Job drawing, mm, ordinate dimensions from the low corner. One solid piece. Give positions to 0.01 mm unless a question says otherwise; leave off trailing zeros. Order: outer loops, then holes, each group sorted by start corner. A loop starts at its lowest first (then second) coordinate and runs counter-clockwise, first axis right, second up.
Item 1: Band-saw the part on B-B on y = 72. Give the cut face in (x, z).
Item 2: Band-saw the part on C-C on x = 23.5. Give the cut face in (y, z), plus the area to 3 significant figures.
Item 3: Band-saw the part on D-D on z = 2.4. Give the cut face in (x, y).
Item 4: Flat gauge pins, fed straight in: P1, Ø1, axis at y = 25.5, z = 2, coming from the +X side; P2, Ø8, axis at x = 72, y = 72, coming from the -Z side; P3, Ø1.5, axis at y = 30, z = 2, coming from the +X side. Where does each tip first touch, or does it go through?
Item 5: Wall check: L1, parallel to Y at x = 72, z = 1.6; L2, parallel to Y at x = 27.5, z = 1.5; L3, parallel to X at y = 51.5, z = 2.9. Give the ranges that are in metal, low to high.
Item 6: Band-saw the part on A-A on x = 72. Give the cut face in (y, z), plus the area to 3 significant figures.
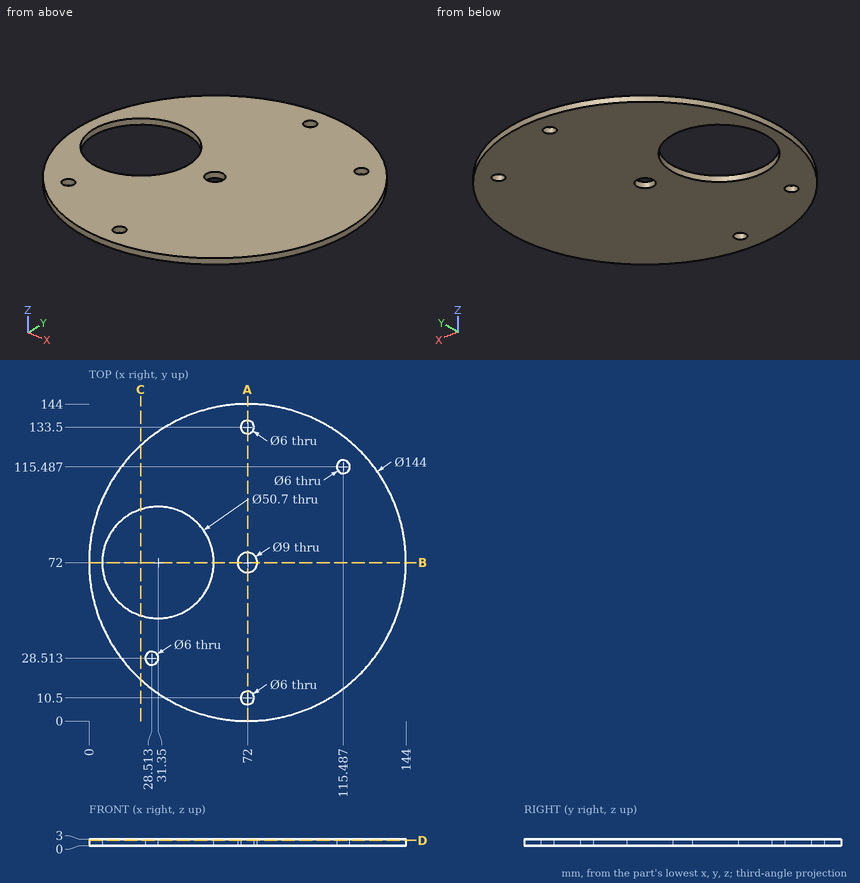
The answers:
1. outline: (0, 0) - (6, 0) - (6, 3) - (0, 3) - close; (56.7, 0) - (67.5, 0) - (67.5, 3) - (56.7, 3) - close; (76.5, 0) - (144, 0) - (144, 3) - (76.5, 3) - close
2. outline: (18.79, 0) - (47.9, 0) - (47.9, 3) - (18.79, 3) - close; (96.1, 0) - (125.21, 0) - (125.21, 3) - (96.1, 3) - close
2. area: 175 mm2
3. outline: circle Ø144 at (72, 72); hole circle Ø50.7 at (31.35, 72); hole circle Ø6 at (28.51, 28.51); hole circle Ø9 at (72, 72); hole circle Ø6 at (72, 10.5); hole circle Ø6 at (72, 133.5); hole circle Ø6 at (115.49, 115.49)
4. P1: stops at x = 127.39
4. P2: passes through
4. P3: stops at x = 131.01
5. L1: y = 0 to 7.5, 13.5 to 67.5, 76.5 to 130.5, 136.5 to 144
5. L2: y = 15.4 to 25.69, 31.34 to 46.94, 97.06 to 128.6
5. L3: x = 2.98 to 16.44, 46.26 to 141.02
6. outline: (0, 0) - (7.5, 0) - (7.5, 3) - (0, 3) - close; (13.5, 0) - (67.5, 0) - (67.5, 3) - (13.5, 3) - close; (76.5, 0) - (130.5, 0) - (130.5, 3) - (76.5, 3) - close; (136.5, 0) - (144, 0) - (144, 3) - (136.5, 3) - close
6. area: 369 mm2
